Print and shaded views of the part. All mm, measured from the part's lowest x, y and z. A direction names the side the tool comes from. Give positions to 0.01 mm unless a question says otherwise; leave off trailing zeros. Write each loop counter-clockwise with the first axis right and the second up, starting at its lowest first coordinate (ties: lowest second). Pieces come first, ordered by that corner, then holes.
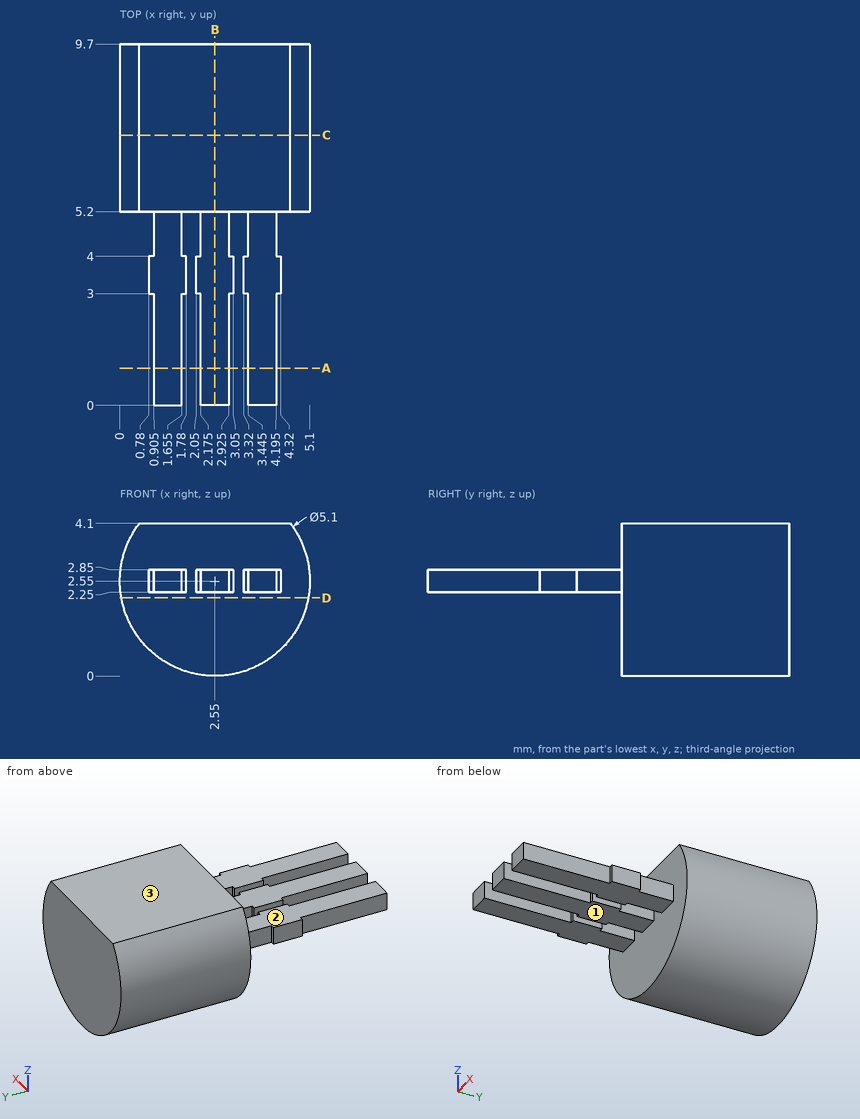
1. 3-axis set-ups, long thin cutter, end or side, ignore diameter. For the marked faces 1, 2 and 3: which of +Z, -Z, +X, -X, +Y, -Y reach the whole face in a straight line?
2. Saw through at A-A on y = 1. Give the cut face in (x, z) (3 decimals), plus the area to 3 significant figures.
3. Saw through at C-C on y = 7.25. Give the cut face in (x, z), plus the area to 3 significant figures.
4. Saw through at D-D on z = 2.1. Give the cut face in (x, y), plus the area to 3 significant figures.
5. Saw through at B-B on x = 2.55. Give the cut face in (y, z).
6. Drill centre lines: line 1 along X through (y, z) = (4.75, 2.65) (3 decimals); line 2 along Y through (x, z) = (1.85, 2.7); line 3 along Z through (x, y) = (2.4, 4). Where is each one in solid material? Low to high.
7. Drop flat-ended pins along their axis: pin 1 (3 mm diameter, centred on x = 1.5, y = 4.5, fed in from -Z); pin 2 (0.7 mm diameter, centred on y = 1.5, z = 2.5, fed in from -X) (3 decimals); pin 3 (2 mm diameter, centred on y = 4.5, z = 3.5, fed in from -X); pin 4 (0.5 mm diameter, centred on y = 3.5, z = 2.5, fed in from +X). Give the stop position or say it passes through.
Outcome:
1. face 1: -Z, +X, -X, -Y
1. face 2: +Z, +X, -X, -Y
1. face 3: +Z, +X, -X, +Y, -Y
2. outline: (0.905, 2.25) - (1.655, 2.25) - (1.655, 2.85) - (0.905, 2.85) - close; (2.175, 2.25) - (2.925, 2.25) - (2.925, 2.85) - (2.175, 2.85) - close; (3.445, 2.25) - (4.195, 2.25) - (4.195, 2.85) - (3.445, 2.85) - close
2. area: 1.35 mm2
3. outline: (0.53, 4.1) arc R2.55 ccw (long way) to (4.57, 4.1) - close
3. area: 17.6 mm2
4. outline: (0.04, 5.2) - (5.06, 5.2) - (5.06, 9.7) - (0.04, 9.7) - close
4. area: 22.6 mm2
5. outline: (0, 2.25) - (5.2, 2.25) - (5.2, 0) - (9.7, 0) - (9.7, 4.1) - (5.2, 4.1) - (5.2, 2.85) - (0, 2.85) - close
6. line 1: x = 0.905 to 1.655, 2.175 to 2.925, 3.445 to 4.195
6. line 2: y = 5.2 to 9.7
6. line 3: z = 2.25 to 2.85
7. pin 1: stops at z = 0
7. pin 2: stops at x = 0.905
7. pin 3: stops at x = 0.01
7. pin 4: stops at x = 4.32
